Part print with two shaded views. Sizes in mm from the minimum x, y, z corner. Round coordinates to 2 decimals unless told otherwise and drop trailing zeros. Write each loop counter-clockwise with the first axis right and the second up, starting at its lowest first coordinate (ties: lowest second). Pieces come first, ordered by that corner, then holes. Notation, with made-up numbers: (-37, 7) - (-18, 7) arc R24 ccw to (-18, 40) - close; hole circle Ø2 at (1, 50). An arc over 180 degrees is marked (long way). Use one line per item in the form item = value. Start each with the question number.
Item 1: Band-saw the part on B-B, the plane z = 1.85. List the corners of the cut face in (x, y).
Item 2: Band-saw the part on A-A, the plane y = 6.95. List the corners of the cut face in (x, z).
Item 3: Drill centre lines: L1, parallel to Y at x = 6.95, z = 2.6; L2, parallel to Z at x = 4.75, y = 6.5. Where is each one in solid material? Low to high.
Item 4: Pull direction Y, two halves, no side cores. Call the marked faces 1, 2 and 3: +Y half, -Y half, draft (parallel to the pull), parting line (faces both ways), or undercut.
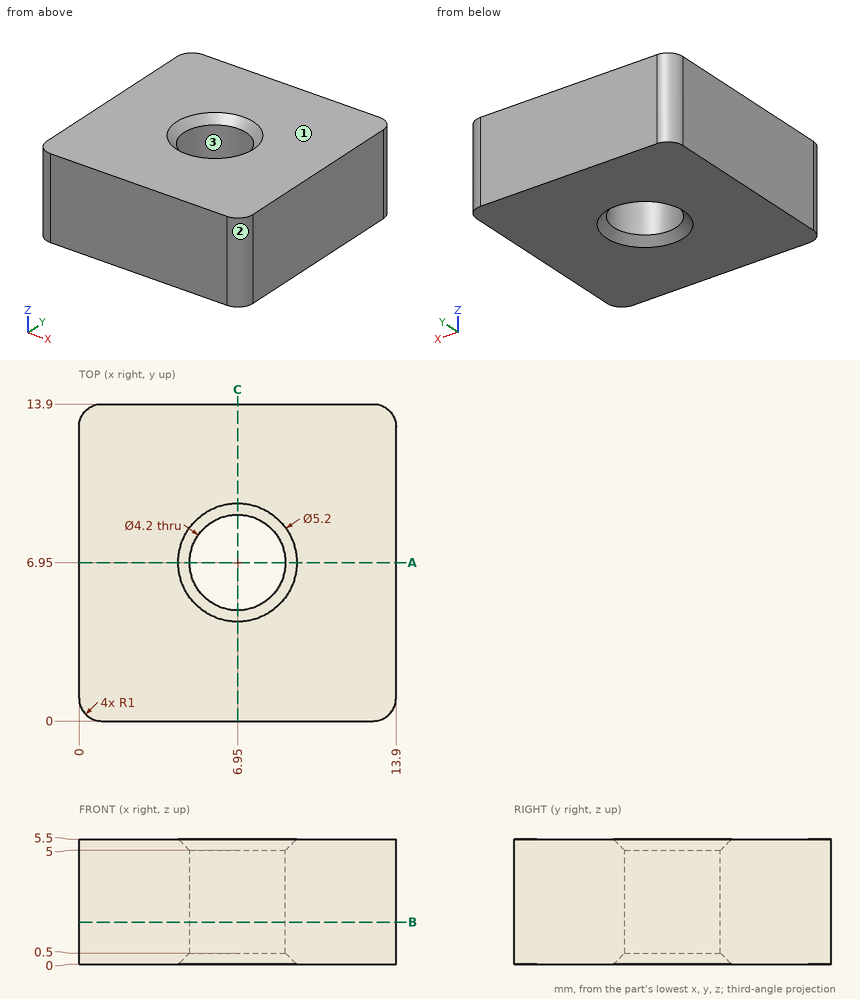
Determined:
q1.outline = (0, 1) arc R1 ccw to (1, 0) - (12.9, 0) arc R1 ccw to (13.9, 1) - (13.9, 12.9) arc R1 ccw to (12.9, 13.9) - (1, 13.9) arc R1 ccw to (0, 12.9) - close; hole circle Ø4.2 at (6.95, 6.95)
q2.outline = (0, 0) - (4.35, 0) - (4.85, 0.5) - (4.85, 5) - (4.35, 5.5) - (0, 5.5) - close; (9.05, 0.5) - (9.55, 0) - (13.9, 0) - (13.9, 5.5) - (9.55, 5.5) - (9.05, 5) - close
q3.L1 = 0 to 4.85, 9.05 to 13.9
q3.L2 = 0.35 to 5.15
q4.face_1 = draft
q4.face_2 = -Y half
q4.face_3 = undercut
